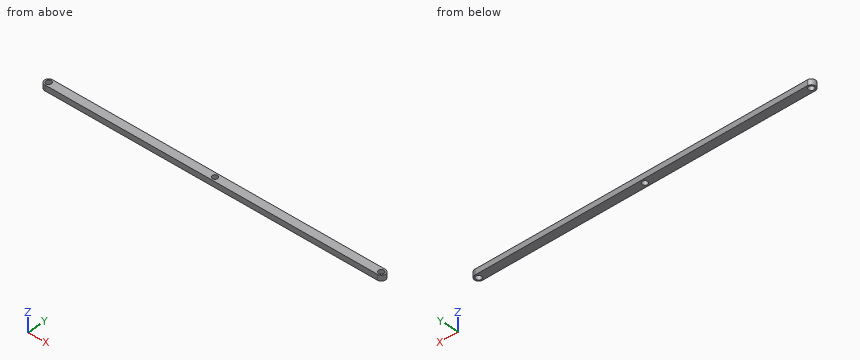
from build123d import *

# Parameters (mm, degrees)
SKETCH2_R           = 1.905
SKETCH2_R_2         = 1.27
BOSS_EXTRUDE1_DEPTH = 2.54


with BuildPart() as part:
    # Sketch2 → Boss-Extrude1 (new body)
    # profile 1 of 5: a face of its own
    with BuildSketch(Plane.XY):
        with BuildLine():
            Line((0, 1.905), (-76.2, 1.905))
            ThreePointArc((-76.2, 1.905), (-74.852961582, 1.347038418), (-74.295, 0))
            ThreePointArc((-74.295, 0), (-74.852961582, -1.347038418), (-76.2, -1.905))
            Line((-76.2, -1.905), (-1.9e-08, -1.905))
            ThreePointArc((-1.9e-08, -1.905), (-1.905, 9e-09), (0, 1.905))
        make_face()
    # profile 2 of 5: a face of its own
    with BuildSketch(Plane.XY):
        with Locations((-76.2, 0)):
            Circle(SKETCH2_R)
        with Locations((-76.2, 0)):
            Circle(SKETCH2_R_2, mode=Mode.SUBTRACT)
    # profile 3 of 5: a face of its own
    with BuildSketch(Plane.XY):
        with BuildLine():
            Line((76.2, 1.905), (0, 1.905))
            ThreePointArc((0, 1.905), (1.347038418, 1.347038418), (1.905, 0))
            ThreePointArc((1.905, 0), (1.347038412, -1.347038425), (-1.9e-08, -1.905))
            Line((-1.9e-08, -1.905), (76.2, -1.905))
            ThreePointArc((76.2, -1.905), (74.295, 0), (76.2, 1.905))
        make_face()
    # profile 4 of 5: a face of its own
    with BuildSketch(Plane.XY):
        with Locations((76.2, 0)):
            Circle(SKETCH2_R)
        with Locations((76.2, 0)):
            Circle(SKETCH2_R_2, mode=Mode.SUBTRACT)
    # profile 5 of 5: a face of its own
    with BuildSketch(Plane.XY):
        Circle(SKETCH2_R)
        Circle(SKETCH2_R_2, mode=Mode.SUBTRACT)
    extrude(amount=BOSS_EXTRUDE1_DEPTH)


solid = part.part
Here's how the part is built. I have some questions about the finished solid (model axes, mm). Coordinates: 2 decimals unless noted, no trailing zeros. Write each loop counter-clockwise with the first axis right and the second up, starting at its lowest first coordinate (ties: lowest second). Pieces come first, ordered by that corner, then holes.
Item 1: I want a section at C-C on z = 1.95. Write out the boundary of the cut face in (x, y) (3 decimals), and give its area (3 significant figures).
Item 2: I want a section at B-B on y = 0. Write out the boundary of the cut face in (x, z) (3 decimals), and give its area (3 significant figures).
Item 3: I want a section at A-A on x = 0. Write out the boundary of the cut face in (y, z) (3 decimals).
Item 4: If I drill on line 1 (X direction, y = -0.15, z = 0.3); line 2 (X direction, y = -0.5, z = 0.5); line 3 (Y direction, x = 0, z = 2.05) (3 decimals), over which ranges is the centre line in solid material (lowest first)?
Findings below:
1. outline: (-76.2, -1.905) - (76.2, -1.905) arc R1.905 ccw to (76.2, 1.905) - (-76.2, 1.905) arc R1.905 ccw to start; hole circle Ø2.54 at (-76.2, 0); hole circle Ø2.54 at (0, 0); hole circle Ø2.54 at (76.2, 0)
1. area: 577 mm2
2. outline: (-78.105, 0) - (-77.47, 0) - (-77.47, 2.54) - (-78.105, 2.54) - close; (-74.93, 0) - (-1.27, 0) - (-1.27, 2.54) - (-74.93, 2.54) - close; (1.27, 0) - (74.93, 0) - (74.93, 2.54) - (1.27, 2.54) - close; (77.47, 0) - (78.105, 0) - (78.105, 2.54) - (77.47, 2.54) - close
2. area: 377 mm2
3. outline: (-1.905, 0) - (-1.27, 0) - (-1.27, 2.54) - (-1.905, 2.54) - close; (1.27, 0) - (1.905, 0) - (1.905, 2.54) - (1.27, 2.54) - close
4. line 1: x = -78.1 to -77.46, -74.94 to -1.26, 1.26 to 74.94, 77.46 to 78.1
4. line 2: x = -78.04 to -77.37, -75.03 to -1.17, 1.17 to 75.03, 77.37 to 78.04
4. line 3: y = -1.905 to -1.27, 1.27 to 1.905
